Build history of the part. All positions in model axes, mm. Face numbers are marked on the shaded views. A direction names the side the tool comes from. Coordinates: 2 decimals unless noted, no trailing zeros. Order: outer loops, then holes, each group sorted by start corner. A loop starts at its lowest first (then second) coordinate and runs counter-clockwise, first axis right, second up. Notation, with made-up numbers: M -25.5,45.5 L 9.5,45.5 A21 cw 9.5,64.5 Z; hole C 81.5,45 d2. An arc over 180 degrees is marked long. Write item = value, one per line. Start each with the question number.
Q1. Drill centre lines: probe 1 along X at (y, z) = (2, 30); probe 2 along X at (y, z) = (2.8, -30); probe 3 along Z at (x, y) = (7.5, 27.5). Where is each one in solid material? Low to high.
Q2. Pull direction X, two halves, no side cores. Call the marked faces 1, 2, 3 and 4: released by +X, released by -X, zero draft, split by the parting line, or undercut.
Q3. Band-saw the part on A-A on y = 3.5. Write the cut outline in (x, z).
Q4. Band-saw the part on B-B on z = 34. Write the cut outline in (x, y).
Q5. Band-saw the part on C-C on x = 0. Write the cut outline in (y, z).
Q6. Pin check, flat tips, straight feed: P1, Ø6, axis at y = 28, z = 33, coming from the -X side; P2, Ø1.5, axis at x = 12.5, y = 3.5, coming from the +Z side; P3, Ø3, axis at y = 28, z = 33, coming from the -X side; P4, Ø6, axis at x = -30, z = -30, coming from the +Y side. Stop position of each tip, or through.
Q7. 3-axis set-ups, long thin cutter, end or side, ignore diameter. For the marked faces 5 and 6: which of +Z, -Z, +X, -X, +Y, -Y reach the whole face in a straight line?
Q8. Band-saw the part on D-D on y = 24. Write the cut outline in (x, z).
```python
from build123d import *

# Parameters (mm, degrees)
BOSS_EXTRUDE1_DEPTH     = 5
SKETCH2_R               = 30
BOSS_EXTRUDE2_DEPTH     = 3
SKETCH3_R               = 27.5
BOSS_EXTRUDE3_DEPTH     = 30
SKETCH4_R               = 22.5
CUT_EXTRUDE1_DEPTH      = 69.14690015
SKETCH6_R               = 22.5
CUT_EXTRUDE2_DEPTH      = 69.14690015
CUT_EXTRUDE5_DEPTH      = 69.146900205
CUT_EXTRUDE5_DEPTH_BACK = 13
SKETCH7_W               = 8
SKETCH7_H               = 27.467309478
SKETCH8_W               = 5
SKETCH8_H               = 20
BOSS_EXTRUDE4_DEPTH     = 43
FILLET1_R               = 10
SKETCH9_R               = 2.5
CUT_EXTRUDE6_DEPTH      = 43
SKETCH10_R              = 22.5
CUT_EXTRUDE7_DEPTH      = 43
SKETCH11_R              = 2.5
CUT_EXTRUDE8_DEPTH      = 10


with BuildPart() as part:
    # Sketch1 → Boss-Extrude1 (new body)
    with BuildSketch(Plane(origin=(0, 0, 0), x_dir=(1, 0, 0), z_dir=(0, 1, 0))):
        with BuildLine():
            Line((30, -40), (-30, -40))
            ThreePointArc((-30, -40), (-37.071067812, -37.071067812), (-40, -30))
            Line((-40, -30), (-40, 30))
            ThreePointArc((-40, 30), (-37.071067812, 37.071067812), (-30, 40))
            Line((-30, 40), (30, 40))
            ThreePointArc((30, 40), (37.071067812, 37.071067812), (40, 30))
            Line((40, 30), (40, -30))
            ThreePointArc((40, -30), (37.071067812, -37.071067812), (30, -40))
        make_face()
    extrude(amount=BOSS_EXTRUDE1_DEPTH)

    # Sketch2 → Boss-Extrude2 (add)
    with BuildSketch(Plane(origin=(0, 5, 0), x_dir=(1, 0, 0), z_dir=(0, 1, 0))):
        with Locations(Location((0, 0, 0), (0, 0, 270))):
            Circle(SKETCH2_R)
    extrude(amount=BOSS_EXTRUDE2_DEPTH)

    # Sketch3 → Boss-Extrude3 (add)
    with BuildSketch(Plane(origin=(0, 8, 0), x_dir=(1, 0, 0), z_dir=(0, 1, 0))):
        with Locations(Location((0, 0, 0), (0, 0, 270))):
            Circle(SKETCH3_R)
    extrude(amount=BOSS_EXTRUDE3_DEPTH)

    # Sketch4 → Cut-Extrude1 (cut, through all)
    with BuildSketch(Plane(origin=(0, 38, 0), x_dir=(1, 0, 0), z_dir=(0, 1, 0))):
        with Locations(Location((0, 0, 0), (0, 0, 270))):
            Circle(SKETCH4_R)
    extrude(amount=-CUT_EXTRUDE1_DEPTH, mode=Mode.SUBTRACT)

    # loft up to a face of the part (loft1)
    loft([Face(Wire([part.edges().sort_by_distance((21.869058823, 8, -20.536413178))[0]])), Face(Wire([part.edges().sort_by_distance((-20.046637254, 38, -18.825045413))[0]]))])

    # Sketch6 → Cut-Extrude2 (cut, through all)
    with BuildSketch(Plane(origin=(0, 38, 0), x_dir=(1, 0, 0), z_dir=(0, 1, 0))):
        with Locations(Location((0, 0, 0), (0, 0, 270))):
            Circle(SKETCH6_R)
    extrude(amount=-CUT_EXTRUDE2_DEPTH, mode=Mode.SUBTRACT)

    # Sketch7 → Cut-Extrude5 (cut, two sides: drawn at the far end of the back side and taken through both)
    with BuildSketch(Plane(origin=(0, 0, 0), x_dir=(1, 0, 0), z_dir=(0, 1, 0)).offset(-CUT_EXTRUDE5_DEPTH_BACK)):
        with Locations((0, -26.266345261)):
            Rectangle(SKETCH7_W, SKETCH7_H)
    extrude(amount=CUT_EXTRUDE5_DEPTH + CUT_EXTRUDE5_DEPTH_BACK, mode=Mode.SUBTRACT)

    # Sketch8 → Boss-Extrude4 (add)
    with BuildSketch(Plane.XY):
        with Locations((-6.5, 28)):
            Rectangle(SKETCH8_W, SKETCH8_H)
        with Locations((6.5, 28)):
            Rectangle(SKETCH8_W, SKETCH8_H)
    extrude(amount=BOSS_EXTRUDE4_DEPTH)

    # Fillet1
    fillet1_edges = [part.edges().sort_by_distance(p)[0] for p in [
        (6.5, 18, 43),
        (-6.5, 18, 43),
        (6.5, 38, 43),
        (-6.5, 38, 43),
    ]]
    fillet(fillet1_edges, radius=FILLET1_R - 0.0001)  # a hair under: the kernel refuses the full size

    # Sketch9 → Cut-Extrude6 (cut)
    with BuildSketch(Plane(origin=(9, 0, 0), x_dir=(0, 0, -1), z_dir=(1, 0, 0))):
        with Locations(Location((-33, 28, 0), (0, 0, 90))):
            Circle(SKETCH9_R)
    extrude(amount=-CUT_EXTRUDE6_DEPTH, mode=Mode.SUBTRACT)

    # Sketch10 → Cut-Extrude7 (cut)
    with BuildSketch(Plane(origin=(0, 38, 0), x_dir=(1, 0, 0), z_dir=(0, 1, 0))):
        Circle(SKETCH10_R)
    extrude(amount=-CUT_EXTRUDE7_DEPTH, mode=Mode.SUBTRACT)

    # Sketch11 → Cut-Extrude8 (cut)
    with BuildSketch(Plane(origin=(0, 5, 0), x_dir=(1, 0, 0), z_dir=(0, 1, 0))):
        with Locations(Location((30, -30, 0), (0, 0, 270))):
            Circle(SKETCH11_R)
        with Locations(Location((-30, -30, 0), (0, 0, 270))):
            Circle(SKETCH11_R)
        with Locations(Location((30, 30, 0), (0, 0, 270))):
            Circle(SKETCH11_R)
        with Locations(Location((-30, 30, 0), (0, 0, 270))):
            Circle(SKETCH11_R)
    extrude(amount=-CUT_EXTRUDE8_DEPTH, mode=Mode.SUBTRACT)


solid = part.part
```
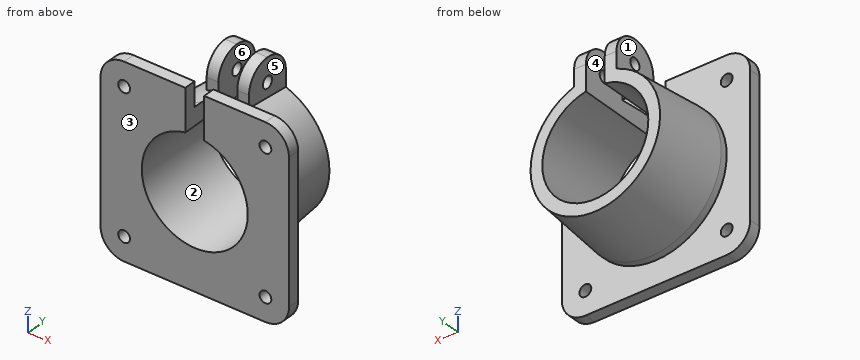
Recorded:
q1.probe_1 = -40 to -32.5, -27.5 to -4, 4 to 27.5, 32.5 to 40
q1.probe_2 = -40 to -32.5, -27.5 to 27.5, 32.5 to 40
q1.probe_3 = -27.37 to -21.21, 21.21 to 30.55, 35.45 to 42.99
q2.face_1 = released by -X
q2.face_2 = undercut
q2.face_3 = zero draft
q2.face_4 = undercut
q3.outline = M -40,-30 A10 ccw -30,-40 L 30,-40 A10 ccw 40,-30 L 40,30 A10 ccw 30,40 L 4,40 L 4,22.14 A22.5 cw long -4,22.14 L -4,40 L -30,40 A10 ccw -40,30 Z; hole C -30,-30 d5; hole C -30,30 d5; hole C 30,-30 d5; hole C 30,30 d5
q4.outline = M -39.17,0 L -4,0 L -4,5 L -39.17,5 Z; M -9,18.05 L -4,18.05 L -4,25.71 L -9,25.71 Z; M -9,30.29 L -4,30.29 L -4,37.95 L -9,37.95 Z; M 4,0 L 39.17,0 L 39.17,5 L 4,5 Z; M 4,18.05 L 9,18.05 L 9,25.71 L 4,25.71 Z; M 4,30.29 L 9,30.29 L 9,37.95 L 4,37.95 Z
q5.outline = M 0,-40 L 5,-40 L 5,-30 L 8,-30 L 38,-27.5 L 38,-22.5 L 0,-22.5 Z
q6.P1 = -9
q6.P2 = 40
q6.P3 = through
q6.P4 = 5
q7.face_5 = +Z, +X, +Y
q7.face_6 = +Z, +Y, -Y
q8.outline = M -9,27.22 A28.67 ccw long 9,27.22 L 9,42.17 L 4,42.17 L 4,22.14 A22.5 cw long -4,22.14 L -4,42.17 L -9,42.17 Z
